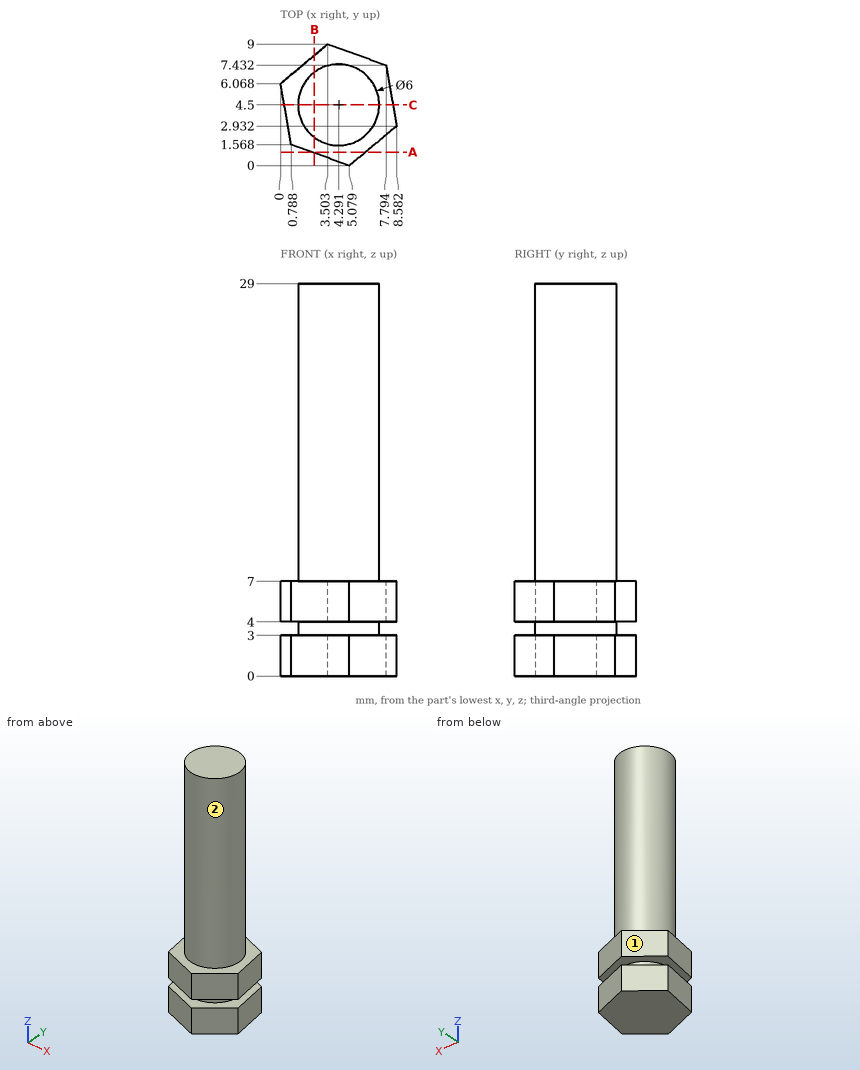
Study the drawing (mm; zero at the part's minimum x, y, z) and answer. A direction names the side the tool comes from. Round coordinates to 2 decimals unless told otherwise and drop trailing zeros. Write each loop counter-clockwise with the first axis right and the second up, starting at its lowest first coordinate (ties: lowest second). Pieces come first, ordered by that corner, then holes. Notation, with made-up numbers: (51, -9.5) -> (84, -9.5) arc R33 ccw to (84, 28.5) -> close; hole circle Ø11 at (-25, 51). An arc over 180 degrees is marked (long way). Answer as CSV lines item,"result". Start each with the question number.
(1) The part is cut by section B-B, the plane x = 2.5. Give the vertices of the cut face in (y, z).
(2) A tool of negligible diameter and unlimited length cuts with its end or side. For the marked faces 1 and 2, from which of +Z, -Z, +X, -X, +Y, -Y can it reach the whole face along a straight path? Write none if from no direction.
(3) The part is cut by section C-C, the plane y = 4.5. Give the vertices of the cut face in (x, z) (1 decimal), then the cut area to 3 significant figures.
(4) Find the intervals of material crossed by probe 1 along Z at (x, y) = (2.5, 7.25); probe 2 along Y at (x, z) = (5, 23.25) (1 decimal); probe 3 along Y at (x, z) = (5.5, 11.75) (1 decimal), in increasing order.
(5) Each of these flat-tipped pins is pushed along its axis until it touches: pin 1 (5 mm diameter, centred on x = 6, z = 15.5, fed in from -Y); pin 2 (4 mm diameter, centred on y = 6, z = 3, fed in from +X) (1 decimal). Where does it stop, or does it pass through?
(6) The part is cut by section A-A, the plane y = 1. Give the vertices of the cut face in (x, z), then the cut area to 3 significant figures.
Output values:
1,outline,"(0.94, 0) -> (8.16, 0) -> (8.16, 3) -> (6.91, 3) -> (6.91, 4) -> (8.16, 4) -> (8.16, 7) -> (6.91, 7) -> (6.91, 29) -> (2.09, 29) -> (2.09, 7) -> (0.94, 7) -> (0.94, 4) -> (2.09, 4) -> (2.09, 3) -> (0.94, 3) -> close"
2,face 1,"+Z, -Z, -X, +Y"
2,face 2,"+Z"
3,outline,"(0.3, 0) -> (8.3, 0) -> (8.3, 3) -> (7.3, 3) -> (7.3, 4) -> (8.3, 4) -> (8.3, 7) -> (7.3, 7) -> (7.3, 29) -> (1.3, 29) -> (1.3, 7) -> (0.3, 7) -> (0.3, 4) -> (1.3, 4) -> (1.3, 3) -> (0.3, 3) -> close"
3,area,"186 mm²"
4,probe 1,"z = 0 to 3, 4 to 7"
4,probe 2,"y = 1.6 to 7.4"
4,probe 3,"y = 1.8 to 7.2"
5,pin 1,"stops at y = 1.5"
5,pin 2,"stops at x = 8.4"
6,outline,"(2.34, 0) -> (6.27, 0) -> (6.27, 3) -> (2.34, 3) -> close; (2.34, 4) -> (6.27, 4) -> (6.27, 7) -> (2.34, 7) -> close"
6,area,"23.6 mm²"
